from build123d import *

# Parameters (mm, degrees)
F0_W           = 41.275
F0_H           = 76.2
F1_DEPTH       = 22.225
F3_D           = 5.6134
F3_CSINK_D     = 10.4394
F3_CSINK_ANGLE = 82
F4_W           = 19.05
F4_H           = 38.1
F5_DEPTH       = 76.201


# Not quite as in the source:
# - a feature names something its author has since deleted; it is built from what else it names


with BuildPart() as f1:
    # F0 (on Right) → F1 (new body)
    with BuildSketch(Plane.YZ):
        Rectangle(F0_W, F0_H)
    extrude(amount=F1_DEPTH)

    # F3 (through all)
    with Locations(Plane.YZ.offset(22.225)):
        with Locations((7.9375, 28.575), (-9.525, -28.575)):
            CounterSinkHole(F3_D / 2, F3_CSINK_D / 2, counter_sink_angle=F3_CSINK_ANGLE)

    # F4 (on face) → F5 (cut, through all)
    with BuildSketch(Plane.XY.offset(38.1)):
        with Locations((9.525, -1.5875)):
            Rectangle(F4_W, F4_H)
    extrude(amount=-F5_DEPTH, mode=Mode.SUBTRACT)


solid = f1.part
Verification items for the finished model (mm, model axes). A direction names the side the tool comes from. Coordinates: 2 decimals unless noted, no trailing zeros. Write each loop counter-clockwise with the first axis right and the second up, starting at its lowest first coordinate (ties: lowest second). Pieces come first, ordered by that corner, then holes. Notation, with made-up numbers: M 30,-3 L 47,-3 A21 ccw 47,21 Z; hole C 54,20.5 d7. An arc over 180 degrees is marked long. One line per question, with ' | ' between items.
1) Sectioned sample at B-B on y = 0. Record the cut outline in (x, z) (3 decimals).
Solutions:
outline: M 19.05,-38.1 L 22.225,-38.1 L 22.225,38.1 L 19.05,38.1 Z
2) Sectioned sample at C-C on x = 15. Record the cut outline in (y, z).
Solutions:
outline: M 17.46,-38.1 L 20.64,-38.1 L 20.64,38.1 L 17.46,38.1 Z
3) Release check for a two-part mould opening along Z. For faces 1 (the face through (9, 17.463, 1)), 2 (the face through (19.3, 4.5, -38.1)), 3 (the face through (19.58, -9.14, -25.68)) record: +Z half, -Z half, draft (parallel to the pull), parting line (faces both ways), or undercut.
Solutions:
face 1: draft | face 2: -Z half | face 3: undercut
4) Access from +Z, -Z, +X, -X, +Y, -Y to the whole of each face (thin tool, end or side, straight path). Record for faces 4 (the face through (19.58, 8.32, 31.47)), 5 (the face through (19.05, -2, 1)).
Solutions:
face 4: +X | face 5: +Z, -Z, -X, -Y
5) Depth check by flat-ended pin: pin 1 Ø4 at (y, z) = (-2.5, -9.5) entering from -X; pin 2 Ø9 at (y, z) = (7.94, 28.58) entering from +X. Enter the tip coordinate at first touch or a pass-through.
Solutions:
pin 1: x = 19.05 | pin 2: x = 21.4
6) Material ranges on L1, parallel to X at y = -5.5, z = 8.5 (3 decimals); L2, parallel to Y at x = 5.75, z = 7, recorded low to high.
Solutions:
L1: 19.05 to 22.225 | L2: 17.46 to 20.64
